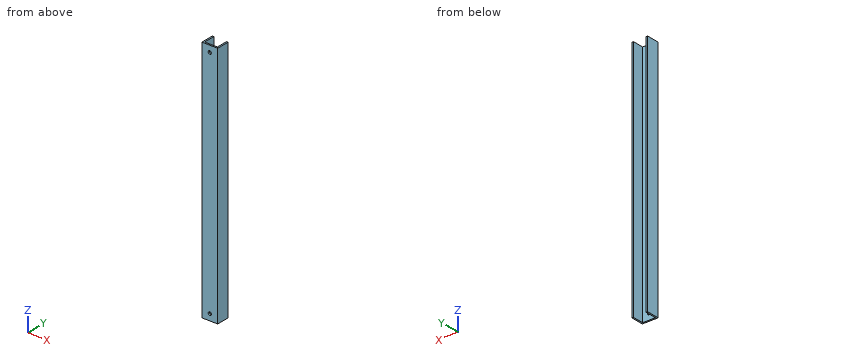
Autodesk Inventor part; units mm, degrees
ref_plane "YZ Plane" through (0, 0, 0) normal (1, 0, 0) x (0, 1, 0)
ref_plane "XZ Plane" through (0, 0, 0) normal (0, 1, 0) x (-1, 0, 0)
ref_plane "XY Plane" through (0, 0, 0) normal (0, 0, 1) x (1, 0, 0)
sketch "Sketch1" plane through (0, 0, 0) normal (0, 0, 1) x (1, 0, 0)
  line L0 (-15.7, 12.7) -> (-12.7, 12.7)
  line L1 (-12.7, 12.7) -> (-12.7, -9.7)
  line L2 (-12.7, -9.7) -> (12.7, -9.7)
  line L3 (12.7, -9.7) -> (12.7, 12.7)
  line L4 (12.7, 12.7) -> (15.7, 12.7)
  line L5 (15.7, 12.7) -> (15.7, -12.7)
  line L6 (15.7, -12.7) -> (-15.7, -12.7)
  line L7 (-15.7, -12.7) -> (-15.7, 12.7)
  point P0 (0, 0)
  dimension "d0" = 3
  dimension "d2" = 3
  dimension "d3" = 25.4
  dimension "d4" = 31.4
  dimension "d5" = 15.7
  dimension "d7" = 12.7
  dimension "d8" = 3
extrude "Extrusion1" add sketch "Sketch1" against normal blind 482.6
sketch "Sketch3" plane through (-12.7, -9.7, 0) normal (0, 1, 0) x (1, 0, 0)
  line L0 (0, 0) -> (25.4, 0)
  line L1 (25.4, 0) -> (25.4, 482.6)
  line L2 (0, 482.6) -> (25.4, 482.6)
  line L3 (0, 0) -> (0, 482.6)
  line L4 (0, 0) -> (0, 25.4) construction
  line L5 (0, 25.4) -> (25.4, 25.4) construction
  line L6 (25.4, 25.4) -> (25.4, 0) construction
  line L7 (25.4, 0) -> (0, 0) construction
  line L8 (12.7, 0) -> (12.7, 25.4) construction
  line L9 (0, 12.7) -> (25.4, 12.7) construction
  line L10 (0, 482.6) -> (25.4, 482.6) construction
  line L11 (25.4, 482.6) -> (25.4, 457.2) construction
  line L12 (25.4, 457.2) -> (0, 457.2) construction
  line L13 (0, 457.2) -> (0, 482.6) construction
  line L14 (12.7, 457.2) -> (12.7, 482.6) construction
  line L15 (0, 469.9) -> (25.4, 469.9) construction
  circle A0 centre (12.7, 469.9) radius 3.175
  circle A1 centre (12.7, 12.7) radius 3.175
  dimension "d15" = 25.4
  dimension "d16" = 25.4
  dimension "d17" = 6.35
  dimension "d18" = 6.35
extrude "Extrusion3" cut sketch "Sketch3" against normal blind 10 contours A0 | A1
equation "\"d2\" = d0"
equation "\"d8\" = d0"
properties part number "19in c-channel"
Geometry: final body of the model. Coordinates: model frame, mm. Give positions to 0.01 mm unless a question says otherwise; leave off trailing zeros. Loops run counter-clockwise (first coordinate to the right, second up) from the corner with the lowest first, then second, coordinate; pieces in that order, holes last. Notation, with made-up numbers: (87.25, 34.5) -> (96.25, 34.5) arc R9 ccw to (96.25, 45.5) -> close; hole circle Ø2 at (63.5, 12). An arc over 180 degrees is marked (long way). Put each result on its own line as item: value.
1. Ray query, line 1 along Z through (x, y) = (0, -11.6) (3 decimals); line 2 along X through (y, z) = (-3.75, -360.5); line 3 along X through (y, z) = (-11.15, -12.7) (3 decimals). Return the intervals inside material, ascending. Write a range as [from, to].
Taken from the geometry:
line 1: z = [-482.6, -473.075], [-466.725, -15.875], [-9.525, 0]
line 2: x = [-15.7, -12.7], [12.7, 15.7]
line 3: x = [-15.7, -3.175], [3.175, 15.7]
2. Cut plane B-B (z = -174.5). Return the cut outline in (x, y).
Taken from the geometry:
outline: (-15.7, -12.7) -> (15.7, -12.7) -> (15.7, 12.7) -> (12.7, 12.7) -> (12.7, -9.7) -> (-12.7, -9.7) -> (-12.7, 12.7) -> (-15.7, 12.7) -> close
3. Cut plane C-C (x = 7.5). Return the cut outline in (y, z).
Taken from the geometry:
outline: (-12.7, -482.6) -> (-9.7, -482.6) -> (-9.7, 0) -> (-12.7, 0) -> close
4. Pin query (flat end, axial travel): P1, Ø7.5, axis at x = 0, z = -12.7, coming from the +Y side. Return the tip coordinate at first contact, or that it passes through.
Taken from the geometry:
P1: stops at y = -9.7
5. Cut plane A-A (y = -3). Return the cut outline in (x, z), plus the area to 3 significant figures.
Taken from the geometry:
outline: (-15.7, -482.6) -> (-12.7, -482.6) -> (-12.7, 0) -> (-15.7, 0) -> close; (12.7, -482.6) -> (15.7, -482.6) -> (15.7, 0) -> (12.7, 0) -> close
area: 2,900 mm2
